```python
from build123d import *

# Parameters (mm, degrees)
F1_DEPTH = 50
F3_DEPTH = 10
F5_DEPTH = 4


with BuildPart() as f1:
    # F0 (on Top) → F1 (new body)
    with BuildSketch(Plane.XY):
        Polygon((-65.519929, 8.285898), (-65.519929, 0), (70.430085, 0), (70.430085, 33.757344), (62.757969, 33.757344), (62.757969, 8.285898), align=None)
    extrude(amount=F1_DEPTH)

    # F2 (on face) → F3 (join)
    with BuildSketch(Plane.XZ):
        Polygon((-65.519929, 50), (-65.519929, 46.481945), (-58.691744, 46.481945), (57.310753, 17.327877), (70.430085, 17.327877), (70.430085, 50), align=None)
    extrude(amount=F3_DEPTH)

    # F4 (on face) → F5 (join)
    with BuildSketch(Plane.YZ.offset(70.430085)):
        Polygon((33.757344, 50), (-10, 50), (-10, 17.327877), (0, 17.327877), (33.757344, 17.327877), align=None)
    extrude(amount=F5_DEPTH)


solid = f1.part
```
CAD build for the part. Positions are in the model's coordinates, mm. A direction names the side the tool comes from. Coordinates: 2 decimals unless noted, no trailing zeros. Loops run counter-clockwise (first coordinate to the right, second up) from the corner with the lowest first, then second, coordinate; pieces in that order, holes last. Notation, with made-up numbers: (-3, 9) - (38, 9) arc R26 cw to (38, 38) - close; hole circle Ø10 at (-24, -24.75). An arc over 180 degrees is marked (long way). Use CSV: the item, a comma, the result in double quotes. Start each with the question number.
Q1. Probe probe 1 along X at (y, z) = (31.5, 6.5); probe 2 along Y at (x, z) = (43.5, 42); probe 3 along Y at (x, z) = (41.5, 4). List the from-to ranges inside material, lowest first. Write a range as from..to.
Q2. Cut at A-A, the plane y = 16. List the corners of the cut face in (x, z).
Q3. Drop flat-ended pins along their axis: P1, Ø1.5, axis at y = 10, z = 9, coming from the +X side; P2, Ø12.5, axis at y = 19, z = 15.5, coming from the -X side; P3, Ø25, axis at x = -24.5, z = 29, coming from the +Y side. Give the stop position or say it passes through.
Q4. Cut at B-B, the plane z = 8.5. List the corners of the cut face in (x, y).
Q5. Cut at D-D, the plane z = 19. List the corners of the cut face in (x, y), then the cut area to 3 significant figures.
Q6. 3-axis set-ups, long thin cutter, end or side, ignore diameter. For faces 1 (the flat face through (70.43, 17, 9)), 2 (the flat face through (62.758, 21, 25)), 3 (the flat face through (-1.5, -4.93, 32.11)): which of +Z, -Z, +X, -X, +Y, -Y reach the whole face in a straight line?
Q7. Cut at C-C, the plane z = 27.5. List the corners of the cut face in (x, y).
Here are the results:
1,probe 1,"62.76..70.43"
1,probe 2,"-10..8.29"
1,probe 3,"0..8.29"
2,outline,"(62.76, 0) - (70.43, 0) - (70.43, 17.33) - (74.43, 17.33) - (74.43, 50) - (62.76, 50) - close"
3,P1,"x = 70.43"
3,P2,"x = 62.76"
3,P3,"y = 8.29"
4,outline,"(-65.52, 0) - (70.43, 0) - (70.43, 33.76) - (62.76, 33.76) - (62.76, 8.29) - (-65.52, 8.29) - close"
5,outline,"(-65.52, 0) - (50.66, 0) - (50.66, -10) - (74.43, -10) - (74.43, 33.76) - (62.76, 33.76) - (62.76, 8.29) - (-65.52, 8.29) - close"
5,area,"1,690 mm2"
6,face 1,"-Z, +X, +Y, -Y"
6,face 2,"+Z, -Z, -X, +Y"
6,face 3,"-Z, -X, -Y"
7,outline,"(-65.52, 0) - (16.84, 0) - (16.84, -10) - (74.43, -10) - (74.43, 33.76) - (62.76, 33.76) - (62.76, 8.29) - (-65.52, 8.29) - close"
